```python
from build123d import *

# Parameters (mm, degrees)
SKETCH1_R           = 18.4
BOSS_EXTRUDE1_DEPTH = 26.5
SKETCH2_R           = 17.4
BOSS_EXTRUDE2_DEPTH = 30.7
SKETCH3_R           = 6
BOSS_EXTRUDE3_DEPTH = 6.5
SKETCH4_R           = 3
BOSS_EXTRUDE4_DEPTH = 15.5
CUT_EXTRUDE1_DEPTH  = 14
SKETCH6_R           = 1.5
CUT_EXTRUDE2_DEPTH  = 8


with BuildPart() as part:
    # Sketch1 → Boss-Extrude1 (new body)
    with BuildSketch(Plane.XY.offset(26.5)):
        Circle(SKETCH1_R)
    extrude(amount=-BOSS_EXTRUDE1_DEPTH)

    # Sketch2 → Boss-Extrude2 (add)
    with BuildSketch(Plane.XY):
        Circle(SKETCH2_R)
    extrude(amount=-BOSS_EXTRUDE2_DEPTH)

    # Sketch3 → Boss-Extrude3 (add)
    with BuildSketch(Plane.XY.offset(26.5)):
        with Locations(Location((0, -7, 0), (0, 0, 180))):
            Circle(SKETCH3_R)
    extrude(amount=BOSS_EXTRUDE3_DEPTH)

    # Sketch4 → Boss-Extrude4 (add)
    with BuildSketch(Plane.XY.offset(33)):
        with Locations((0, -7)):
            Circle(SKETCH4_R)
    extrude(amount=BOSS_EXTRUDE4_DEPTH)

    # Sketch5 → Cut-Extrude1 (cut)
    with BuildSketch(Plane.XY.offset(48.5)):
        Polygon((-4.411433232, -4.6), (4.412869288, -4.6), (0, -0.417886065), align=None)
    extrude(amount=-CUT_EXTRUDE1_DEPTH, mode=Mode.SUBTRACT)

    # Sketch6 → Cut-Extrude2 (cut)
    with BuildSketch(Plane.XY.offset(26.5)):
        with Locations((-15.5, 0)):
            Circle(SKETCH6_R)
        with Locations((-7.75, 13.423393759)):
            Circle(SKETCH6_R)
        with Locations((7.75, 13.423393759)):
            Circle(SKETCH6_R)
        with Locations((15.5, 0)):
            Circle(SKETCH6_R)
        with Locations((7.75, -13.423393759)):
            Circle(SKETCH6_R)
        with Locations((-7.75, -13.423393759)):
            Circle(SKETCH6_R)
    extrude(amount=-CUT_EXTRUDE2_DEPTH, mode=Mode.SUBTRACT)


solid = part.part
```
Geometry check sheet. Reference: the model listing, model coordinates, mm. A direction names the side the tool comes from. Coordinates: 2 decimals unless noted, no trailing zeros. Order: outer loops, then holes, each group sorted by start corner. A loop starts at its lowest first (then second) coordinate and runs counter-clockwise, first axis right, second up. Notation, with made-up numbers: M 15,17.5 L 65,17.5 A31 cw 65,48.5 Z; hole C 54,65.5 d7. An arc over 180 degrees is marked long. One line per question, with ' | ' between items. Start each with the question number.
Item 1: Draft check along X on faces 4 (the cylindrical face through (-17, 0, 23)), 5 (the cylindrical face through (-3.772, -16.986, -15.135)), 6 (the flat face through (0, -7, 48.5)). Enter one of: pulls with the +X half, pulls with the -X half, needs draft (parallel to the pull), parting line crosses it, or undercut.
Item 2: Material ranges on L1, parallel to X at y = 0.5, z = 25; L2, parallel to Z at x = -10, y = 2; L3, parallel to Z at x = 5.5, y = -17, recorded low to high. Write a range as [from, to].
Item 3: Cross-section at A-A on x = 0. Enter the section's corners in (y, z), then the cut area to 3 significant figures.
Item 4: Cross-section at C-C on z = -7. Enter the section's corners in (x, y), then the cut area to 3 significant figures.
Item 5: Cross-section at B-B on y = 0. Enter the section's corners in (x, z), then the cut area to 3 significant figures.
Item 6: Gauge pin test, flat ends, axial feed: pin 1 (1.8 mm diameter, centred on x = 0, z = 42, fed in from +Y); pin 2 (1.5 mm diameter, centred on x = 16, y = -0.5, fed in from +Z); pin 3 (6 mm diameter, centred on x = 5, y = 4, fed in from +Z). Record the tip position at first contact, or that the pin passes through.
Item 7: Set-up check for faces 1 (the flat face through (14, 11, 0)), 2 (the cylindrical face through (14, 0, 23)), 3 (the flat face through (0, 0, -30.7)): record each of +Z, -Z, +X, -X, +Y, -Y from which the full face is reachable in a straight line by a thin tool's end or side.
Item 8: Cross-section at D-D on x = 7.75. Enter the section's corners in (y, z), then the cut area to 3 significant figures.
Findings:
1) face 4: undercut | face 5: parting line crosses it | face 6: needs draft
2) L1: x = [-18.39, -16.91], [-14.09, 14.09], [16.91, 18.39] | L2: z = [-30.7, 26.5] | L3: z = [0, 26.5]
3) outline: M -18.4,0 L -17.4,0 L -17.4,-30.7 L 17.4,-30.7 L 17.4,0 L 18.4,0 L 18.4,26.5 L -1,26.5 L -1,33 L -4,33 L -4,34.5 L -4.6,34.5 L -4.6,48.5 L -10,48.5 L -10,33 L -13,33 L -13,26.5 L -18.4,26.5 Z | area: 2,210 mm²
4) outline: C 0,0 d34.8 | area: 951 mm²
5) outline: M -18.4,0 L -17.4,0 L -17.4,-30.7 L 17.4,-30.7 L 17.4,0 L 18.4,0 L 18.4,26.5 L 17,26.5 L 17,18.5 L 14,18.5 L 14,26.5 L -14,26.5 L -14,18.5 L -17,18.5 L -17,26.5 L -18.4,26.5 Z | area: 2,000 mm²
6) pin 1: stops at y = -4.6 | pin 2: stops at z = 18.5 | pin 3: stops at z = 26.5
7) face 1: -Z | face 2: +Z | face 3: -Z, +X, -X, +Y, -Y
8) outline: M -16.69,0 L -15.58,0 L -15.58,-30.7 L 15.58,-30.7 L 15.58,0 L 16.69,0 L 16.69,26.5 L 14.92,26.5 L 14.92,18.5 L 11.92,18.5 L 11.92,26.5 L -11.92,26.5 L -11.92,18.5 L -14.92,18.5 L -14.92,26.5 L -16.69,26.5 Z | area: 1,790 mm²
